The model under review builds one solid part; all positions refer to its coordinate system, in mm. A direction names the side the tool comes from. Round coordinates to 2 decimals unless told otherwise and drop trailing zeros. Order: outer loops, then holes, each group sorted by start corner. A loop starts at its lowest first (then second) coordinate and runs counter-clockwise, first axis right, second up.
1) Consider section B-B (z = 39.5). Give the boundary of the cut face in (x, y).
2) Consider section C-C (x = 54). Give the boundary of the cut face in (y, z).
3) Machinability: for faces 4 (the face through (67.93, 2.46, 38.88)), 5 (the face through (54, 15, 37)), which of the approach directions +Z, -Z, +X, -X, +Y, -Y give a long, thin tool a straight path to every point of the face, cutting with its end or side? Answer none if there is none.
4) Consider section A-A (y = 1.75). Give the boundary of the cut face in (x, z).
5) Clearance check with flat-ended pins moving along their axes: P1, Ø1.5, axis at y = 3, z = 29, coming from the +X side; P2, Ø1.5, axis at y = 2, z = 29.5, coming from the -X side; P3, Ø10.5, axis at x = 55, z = 36, coming from the -Y side; P4, Ø3, axis at y = 11.5, z = 48.5, coming from the +X side. State where each tip first meets the part, or that it passes through.
6) To check wall thickness, follow L1, parallel to Z at x = 54, y = 1.5; L2, parallel to X at y = 1.5, z = 41.75; L3, parallel to Z at x = 64.5, y = 1.25. State the ranges of each line that lie inside material, in increasing order.
7) Consider section D-D (y = 9). Give the boundary of the cut face in (x, z), then the cut area to 3 significant figures.
8) Mouldability with a two-part tool opening along X and no side actions: class faces 1 (the face through (53, 5, 36.7)), 2 (the face through (54, 0, 39)), 3 (the face through (67.982, 7.395, 41.431)) as pulls with the +X half, pulls with the -X half, needs draft (parallel to the pull), parting line crosses it, or undercut.
Solid Edge part; units mm, degrees
sketch "Sketch1" plane through (0, 0, 0) normal (0, -1, 0) x (1, 0, 0)
  circle A0 centre (53.6751, 36.9251) radius 15
extrude "ExtrudedProtrusion_1" add sketch "Sketch1" against normal blind 15
sketch "Sketch2" plane through (63.9305, 0, 41.9251) normal (0, -1, 0) x (1, 0, 0)
  line L0 (-8, -10) -> (-8, -15)
  arc A0 (-8, -15) -> (-12, -15) centre (-10, -15) cw
  line L1 (-12, -15) -> (-12, -10)
  arc A1 (-12, -10) -> (-17, -5) centre (-17, -10) ccw
  line L2 (-17, -5) -> (-22, -5)
  arc A2 (-22, -5) -> (-22, -1) centre (-22, -3) cw
  line L3 (-22, -1) -> (-17, -1)
  arc A3 (-17, -1) -> (-14, 2) centre (-17, 2) ccw
  arc A4 (-14, 2) -> (-6, 2) centre (-10, -2.5133) cw
  arc A5 (-3, -1) -> (-6, 2) centre (-3, 2) cw
  line L4 (2, -1) -> (-3, -1)
  arc A6 (2, -5) -> (2, -1) centre (2, -3) ccw
  line L5 (-3, -5) -> (2, -5)
  arc A7 (-8, -10) -> (-3, -5) centre (-3, -10) cw
  dimension "D1" = 8
  dimension "D2" = 12
  dimension "D3" = 3
  dimension "D4" = 17
  dimension "D5" = 22
  dimension "D6" = 2
extrude "Cutout1" cut sketch "Sketch2" against normal blind 5
sketch "Sketch3" plane through (63.9305, 5, 35.4251) normal (0, -1, 0) x (1, 0, 0)
  circle A0 centre (-10, 3.5) radius 2.25
extrude "ExtrudedProtrusion_3" add sketch "Sketch3" along normal blind 5
Answer below:
1. outline: (38.9, 0) - (40.01, 0) - (40.01, 5) - (51.76, 5) - (51.76, 0) - (56.11, 0) - (56.11, 5) - (67.85, 5) - (67.85, 0) - (68.45, 0) - (68.45, 15) - (38.9, 15) - close
2. outline: (0, 21.93) - (15, 21.93) - (15, 51.92) - (0, 51.92) - (0, 45.44) - (5, 45.44) - (5, 41.17) - (0, 41.17) - (0, 36.68) - (5, 36.68) - (5, 24.93) - (0, 24.93) - close
3. face 4: -Y
3. face 5: +Z, -Z, +X, -X, +Y
4. outline: circle Ø30 at (53.68, 36.93); circle Ø4.5 at (53.93, 38.93); hole (41.93, 36.93) - (46.93, 36.93) arc R5 cw to (51.93, 31.93) - (51.93, 26.93) arc R2 ccw to (55.93, 26.93) - (55.93, 31.93) arc R5 cw to (60.93, 36.93) - (65.93, 36.93) arc R2 ccw to (65.93, 40.93) - (60.93, 40.93) arc R3 cw to (57.93, 43.93) arc R6.03 ccw to (49.93, 43.93) arc R3 cw to (46.93, 40.93) - (41.93, 40.93) arc R2 ccw to start
5. P1: stops at x = 66.85
5. P2: stops at x = 40.24
5. P3: stops at y = 0
5. P4: stops at x = 64.79
6. L1: z = 21.93 to 24.93, 36.68 to 41.17, 45.44 to 51.92
6. L2: x = 39.47 to 49, 58.86 to 67.88
6. L3: z = 26.54 to 36.93, 40.93 to 47.31
7. outline: circle Ø30 at (53.68, 36.93)
7. area: 707 mm2
8. face 1: undercut
8. face 2: needs draft
8. face 3: parting line crosses it
